Could you check a few things on this drawing? It's one solid part, dimensions in mm from its lowest x, y, z. Give positions to 0.01 mm unless a question says otherwise; leave off trailing zeros. Write each loop counter-clockwise with the first axis right and the second up, starting at its lowest first coordinate (ties: lowest second). Pieces come first, ordered by that corner, then holes.
1. I'm going to push flat-ended pins straight in: pin 1 (0.6 mm diameter, centred on y = 1.5, z = 3, fed in from +X); pin 2 (1 mm diameter, centred on y = 1.5, z = 10.5, fed in from -X). Where does each tip first touch, or does it pass through?
2. Suppose I cut it at C-C (z = 18.5). Please give me the cut outline in (x, y), and give its area (3 significant figures).
3. If I drill on probe 1 along X at (y, z) = (1.95, 50.5); probe 2 along Z at (x, y) = (24, 1.15); probe 3 along Z at (x, y) = (17.5, 1.3), over which ranges is the centre line in solid material (lowest first)?
4. Suppose I cut it at A-A (z = 28). Please give me the cut outline in (x, y).
5. Suppose I cut it at B-B (y = 0.6). Give the number of separate pieces and of enclosed holes in the cut face, and give its area (3 significant figures).
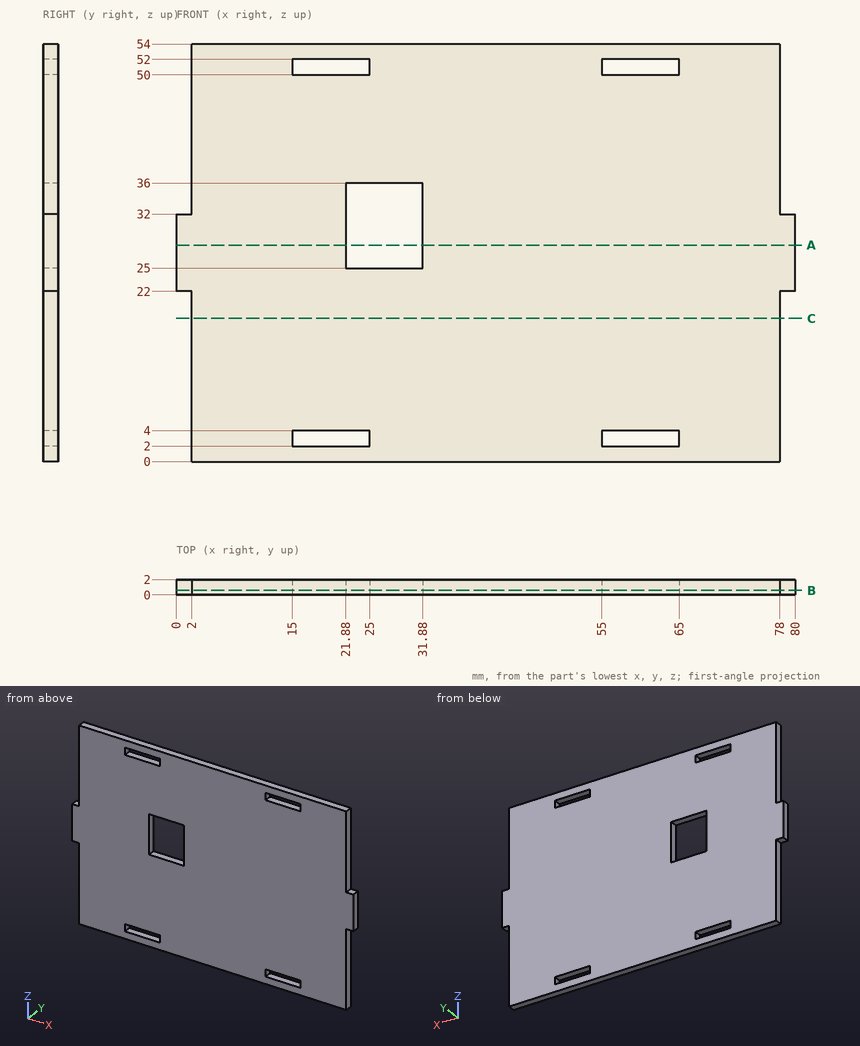
Checks:
1. pin 1: stops at x = 78
1. pin 2: stops at x = 2
2. outline: (2, 0) - (78, 0) - (78, 2) - (2, 2) - close
2. area: 152 mm2
3. probe 1: x = 2 to 15, 25 to 55, 65 to 78
3. probe 2: z = 0 to 2, 4 to 25, 36 to 50, 52 to 54
3. probe 3: z = 0 to 2, 4 to 50, 52 to 54
4. outline: (0, 0) - (21.88, 0) - (21.88, 2) - (0, 2) - close; (31.88, 0) - (80, 0) - (80, 2) - (31.88, 2) - close
5. separate pieces: 1
5. enclosed holes: 5
5. area: 3,950 mm2
